from build123d import *

# Parameters (mm, degrees)
CROQUIS1_R                                     = 2.5
SALIENTE_EXTRUIR1_DEPTH                        = 8
PERFORADOR_PARA_ROSCAR_PARA_MACHO_DE_ROS_D     = 2.05
PERFORADOR_PARA_ROSCAR_PARA_MACHO_DE_ROS_DEPTH = 10
PERFORADOR_PARA_ROSCAR_PARA_MACHO_DE_ROS_TIP   = 0.615882135


with BuildPart() as part:
    # Croquis1 → Saliente-Extruir1 (new body)
    with BuildSketch(Plane.XY):
        with BuildLine():
            Line((-51.94164691, 0), (-19.94164691, 0))
            Line((-19.94164691, 0), (-19.94164691, 4))
            Line((-19.94164691, 4), (-29.94164691, 4))
            ThreePointArc((-29.94164691, 4), (-35.94164691, 10), (-41.94164691, 4))
            Line((-41.94164691, 4), (-51.94164691, 4))
            Line((-51.94164691, 4), (-51.94164691, 0))
        make_face()
        with Locations((-35.94164691, 4)):
            Circle(CROQUIS1_R, mode=Mode.SUBTRACT)
    extrude(amount=SALIENTE_EXTRUIR1_DEPTH)

    # Perforador para roscar para macho de roscar para M2.5x0.451
    with Locations(Plane(origin=(0, 4, 0), x_dir=(1, 0, 0), z_dir=(0, 1, 0))):
        with Locations((-46.940104762, -5.012552849), (-24.941517603, -5.012552849)):
            Hole(PERFORADOR_PARA_ROSCAR_PARA_MACHO_DE_ROS_D / 2, depth=PERFORADOR_PARA_ROSCAR_PARA_MACHO_DE_ROS_DEPTH)
            with Locations((0, 0, -(PERFORADOR_PARA_ROSCAR_PARA_MACHO_DE_ROS_DEPTH + PERFORADOR_PARA_ROSCAR_PARA_MACHO_DE_ROS_TIP / 2))):  # 118° drill point
                Cone(0, PERFORADOR_PARA_ROSCAR_PARA_MACHO_DE_ROS_D / 2, PERFORADOR_PARA_ROSCAR_PARA_MACHO_DE_ROS_TIP, mode=Mode.SUBTRACT)


solid = part.part
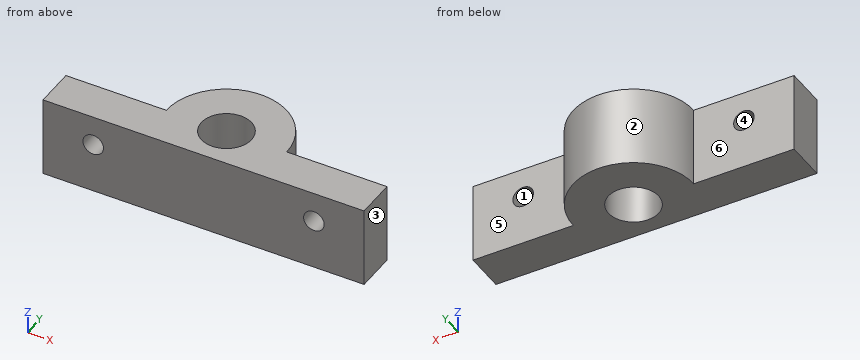
The model under review builds one solid part; all positions refer to its coordinate system, in mm. Face numbers are marked on the shaded views. A direction names the side the tool comes from. Coordinates: 2 decimals unless noted, no trailing zeros. Loops run counter-clockwise (first coordinate to the right, second up) from the corner with the lowest first, then second, coordinate; pieces in that order, holes last. Notation, with made-up numbers: M 85.5,2 L 115.5,2 A15 ccw 115.5,13 Z; hole C 11,87.5 d4. An arc over 180 degrees is marked long. Put each result on its own line as item: value. Start each with the question number.
Q1. Add section B-B (z = 1). Write out the cut boundary in (x, y).
Q2. Add section D-D (x = -22.5). Write out the cut boundary in (y, z).
Q3. Add section A-A (y = 4.5). Write out the cut boundary in (x, z).
Q4. Add section C-C (y = 3). Write out the cut boundary in (x, z) (3 decimals).
Q5. The part is to be moulded in two halves that separate along X. For the marked faces 1, 2 and 3, say which applies: +X half, -X half, draft (parallel to the pull), parting line (faces both ways), or undercut.
Q6. Clearance check with a flat-ended pin moving along its axis: pin 1 (3.5 mm diameter, centred on x = -24.94, z = 5.01, fed in from +Y). State where the tip first meets the part, or that it passes through.
Q7. For the marked faces 4, 5 and 6, list the 3-axis set-ups (+Z, -Z, +X, -X, +Y, -Y) from which the entire face can be reached by the end or side of a thin tool; tool diameter is ignored.
Q8. Wall thickness on line 1 (Z direction, x = -47, y = 3.5); line 2 (Y direction, x = -42, z = 5.5); line 3 (Y direction, x = -36, z = 0.5): over which ranges is each line inside the solid? List them lowest first.
Answers:
1. outline: M -51.94,0 L -19.94,0 L -19.94,4 L -29.94,4 A6 ccw -41.94,4 L -51.94,4 Z; hole C -35.94,4 d5
2. outline: M 0,0 L 4,0 L 4,8 L 0,8 Z
3. outline: M -41.92,0 L -38.39,0 L -38.39,8 L -41.92,8 Z; M -33.49,0 L -29.96,0 L -29.96,8 L -33.49,8 Z
4. outline: M -51.942,0 L -38.233,0 L -38.233,8 L -51.942,8 Z; M -33.65,0 L -19.942,0 L -19.942,8 L -33.65,8 Z; hole C -46.94,5.013 d2.05; hole C -24.942,5.013 d2.05
5. face 1: undercut
5. face 2: parting line
5. face 3: +X half
6. pin 1: stops at y = 4
7. face 4: +Y, -Y
7. face 5: +Z, -Z, +X, +Y
7. face 6: +Z, -Z, -X, +Y
8. line 1: z = 0 to 3.99, 6.04 to 8
8. line 2: y = 0 to 4
8. line 3: y = 0 to 1.5, 6.5 to 10
